from build123d import *

# Parameters (mm, degrees)
F0_W     = 150
F0_H     = 10
F1_DEPTH = 10
F3_R     = 3.365379
F4_DEPTH = 2
F2_R     = 2.92998
F5_DEPTH = 2


with BuildPart() as f1:
    # F0 (on Front) → F1 (new body)
    with BuildSketch(Plane.XZ):
        with Locations((-0.948794, 5.625204)):
            Rectangle(F0_W, F0_H)
    extrude(amount=F1_DEPTH)

    # F3 (on face) → F4 (join)
    with BuildSketch(Plane.XZ.offset(10)):
        with Locations((6.850945, 4.902036)):
            Circle(F3_R)
    extrude(amount=F4_DEPTH)

    # F2 (on face) → F5 (join)
    with BuildSketch(Plane(origin=(0, 0, 0), x_dir=(-1, 0, 0), z_dir=(0, 1, 0))):
        with Locations((-66.123568, 4.694908)):
            Circle(F2_R)
    extrude(amount=F5_DEPTH)


solid = f1.part
Input: part model. Units: mm. Frame: model coordinates. A direction names the side the tool comes from. Round coordinates to 2 decimals unless told otherwise and drop trailing zeros. Write each loop counter-clockwise with the first axis right and the second up, starting at its lowest first coordinate (ties: lowest second). Pieces come first, ordered by that corner, then holes.
1) Ray query, L1, parallel to Y at x = -49, z = 6; L2, parallel to X at y = -10.75, z = 5; L3, parallel to X at y = 0.25, z = 3. Return the intervals inside material, ascending.
2) Cut plane B-B (x = 32). Return the cut outline in (y, z).
3) Reachability of faces 1 (the flat face through (-75.949, -5, 6)), 2 (the cylindrical face through (4.371, -10.986, 7.177)), 3 (the cylindrical face through (69.05, 0.99, 4.82)) from +Z, -Z, +X, -X, +Y, -Y: full face, straight path, thin tool, end or side. Return the list, or none.
4) Cut plane A-A (x = 7.5). Return the cut outline in (y, z).
5) Contact query for flat-ended pins moving along their axis: P1, Ø5, axis at x = -23, z = 5, coming from the -Y side; P2, Ø5, axis at x = 24, z = 3.5, coming from the +Y side. Output: stop coordinate, or through.
Geometry says:
1. L1: y = -10 to 0
1. L2: x = 3.49 to 10.21
1. L3: x = 63.73 to 68.51
2. outline: (-10, 0.63) - (0, 0.63) - (0, 10.63) - (-10, 10.63) - close
3. face 1: +Z, -Z, -X, +Y, -Y
3. face 2: -Y
3. face 3: +Y
4. outline: (-12, 1.6) - (-10, 1.6) - (-10, 0.63) - (0, 0.63) - (0, 10.63) - (-10, 10.63) - (-10, 8.2) - (-12, 8.2) - close
5. P1: stops at y = -10
5. P2: stops at y = 0
